Source: three-view drawing plus pictorial views. Frame: mm from the lowest corner of the part. A direction names the side the tool comes from. Give positions to 0.01 mm unless a question says otherwise; leave off trailing zeros. Loops run counter-clockwise (first coordinate to the right, second up) from the corner with the lowest first, then second, coordinate; pieces in that order, holes last. Notation, with made-up numbers: (70.5, 16.5) - (124.5, 16.5) arc R13 ccw to (124.5, 38.5) - close; hole circle Ø1 at (13, 10). An arc over 180 degrees is marked (long way). Answer as a JSON object with one key per item and string values.
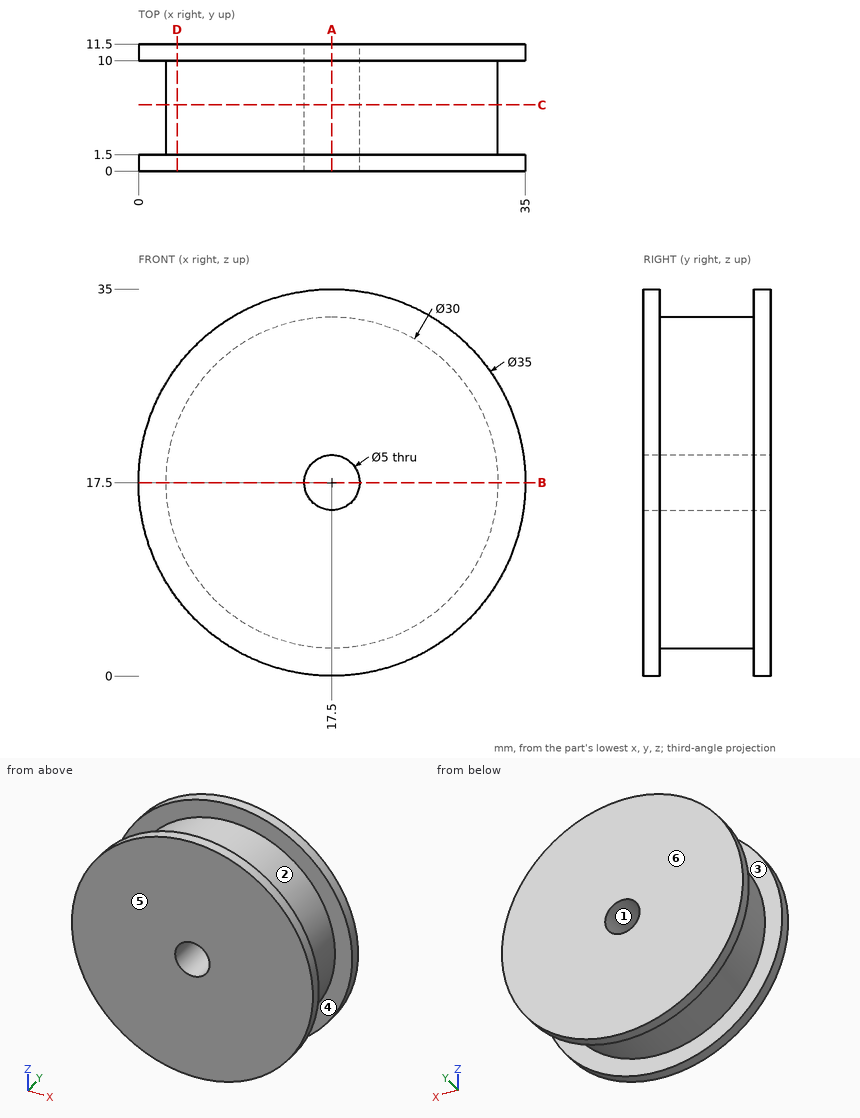
Item 1: Contact query for flat-ended pins moving along their axis: P1, Ø1.5, axis at y = 7.5, z = 9.5, coming from the -X side; P2, Ø3, axis at y = 7, z = 15, coming from the -X side; P3, Ø5, axis at y = 2, z = 13.5, coming from the +X side. Output: stop coordinate, or through.
Geometry check:
{"P1": "stops at x = 4.37", "P2": "stops at x = 2.53", "P3": "stops at x = 34.93"}
Item 2: Access query for the marked faces 1 and 2. Directions: +Z, -Z, +X, -X, +Y, -Y. A direction counts if a zero-diameter tool reaches every point of the face in a straight line with its end or side. Return the directions, or none.
Geometry check:
{"face 1": "+Y, -Y", "face 2": "none"}
Item 3: Cut plane B-B (z = 17.5). Return loops of the section in (x, y), then the cut area to 4 significant figures.
Geometry check:
{"outline": "(0, 0) - (15, 0) - (15, 11.5) - (0, 11.5) - (0, 10) - (2.5, 10) - (2.5, 1.5) - (0, 1.5) - close; (20, 0) - (35, 0) - (35, 1.5) - (32.5, 1.5) - (32.5, 10) - (35, 10) - (35, 11.5) - (20, 11.5) - close", "area": "302.5 mm2"}
Item 4: Cut plane C-C (y = 6). Return loops of the section in (x, z).
Geometry check:
{"outline": "circle Ø30 at (17.5, 17.5); hole circle Ø5 at (17.5, 17.5)"}
Item 5: Cut plane A-A (x = 17.5). Return loops of the section in (y, z).
Geometry check:
{"outline": "(0, 0) - (1.5, 0) - (1.5, 2.5) - (10, 2.5) - (10, 0) - (11.5, 0) - (11.5, 15) - (0, 15) - close; (0, 20) - (11.5, 20) - (11.5, 35) - (10, 35) - (10, 32.5) - (1.5, 32.5) - (1.5, 35) - (0, 35) - close"}
Item 6: Mould query, pull axis Y, two halves, no side actions, for the marked faces 3, 4, 5 and 6. Classes: released by +Y, released by -Y, zero draft, split by the parting line, or undercut.
Geometry check:
{"face 3": "undercut", "face 4": "undercut", "face 5": "released by -Y", "face 6": "released by +Y"}
Item 7: Cut plane D-D (x = 3.5). Return loops of the section in (y, z).
Geometry check:
{"outline": "(0, 7) - (1.5, 7) - (1.5, 12.11) - (10, 12.11) - (10, 7) - (11.5, 7) - (11.5, 28) - (10, 28) - (10, 22.89) - (1.5, 22.89) - (1.5, 28) - (0, 28) - close"}
Item 8: Material intervals for line 1 (X direction, y = 5.75, z = 17.5); line 2 (Y direction, x = 3.5, z = 12); line 3 (X direction, y = 3.75, z = 16), sorted ascending. Write a range as [from, to].
Geometry check:
{"line 1": "x = [2.5, 15], [20, 32.5]", "line 2": "y = [0, 1.5], [10, 11.5]", "line 3": "x = [2.58, 15.5], [19.5, 32.42]"}
